Could you check a few things on this drawing? It's one solid part, dimensions in mm from its lowest x, y, z. A direction names the side the tool comes from. Round coordinates to 2 decimals unless told otherwise and drop trailing zeros. Write each loop counter-clockwise with the first axis right and the second up, starting at its lowest first coordinate (ties: lowest second). Pieces come first, ordered by that corner, then holes. Notation, with made-up numbers: (88.5, 70.25) -> (137.5, 70.25) arc R14 cw to (137.5, 75.25) -> close; hole circle Ø1 at (10.25, -27). An arc over 180 degrees is marked (long way). Answer in a Markdown table with one row per item. Add a question column.
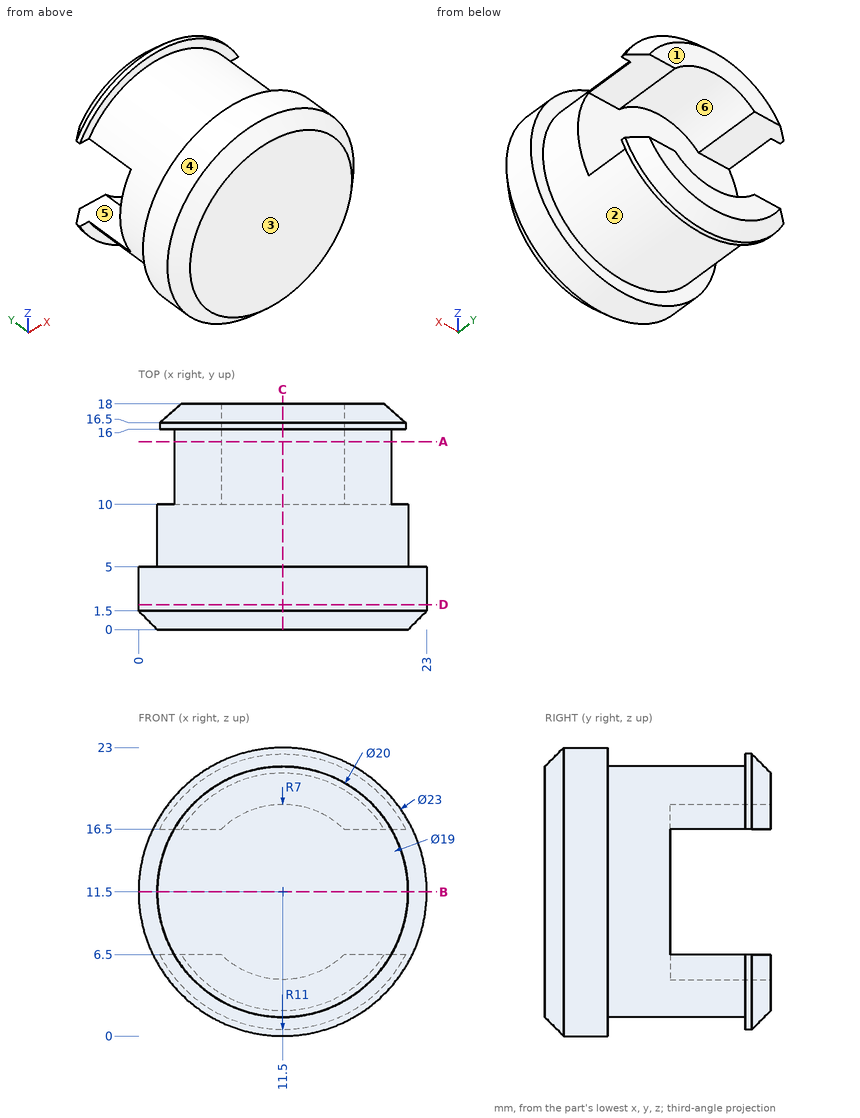
Item 1: If we section it at B-B on z = 11.5: Please give me the cut outline in (x, y), then the cut area to 3 significant figures.
Item 2: On a 3-axis mill with a long thin cutter (end or side, diameter ignored), from which of +Z, -Z, +X, -X, +Y, -Y can I reach the whole of each face in a straight line? I mean the marked faces 4, 5 and 6. Say none if no direction works.
Item 3: If we mould it in two halves opening along Y, with no side actions, what happens to the marked faces 1, 2 and 3? For each: pulls with the +Y half, pulls with the -Y half, needs draft (parallel to the pull), parting line crosses it, or undercut.
Item 4: For P1, Ø2, axis at x = 5, y = 13, coming from the -Z side; P2, Ø5.5, axis at x = 20, y = 13, coming from the -Z side; P3, Ø5.5, axis at x = 18.5, y = 14.5, coming from the +Z side; P4, Ø2, axis at y = 12, z = 10.5, coming from the +X side (3 decimals), each with a flat end and sliding along its axis, tell me the tip position at first contact or that it passes through.
Item 5: If we section it at D-D on y = 2: Please give me the cut outline in (x, z).
Item 6: If we section it at C-C on x = 11.5: Please give me the cut outline in (y, z).
Item 7: I need wall thicknesses on line 1 along X through (y, z) = (8.25, 9.5); line 2 along Y through (x, z) = (3, 18.25); line 3 along Y through (x, z) = (10.25, 12). Which ranges of each line are inside material? Lowest first, please. Write a range as from..to.
Item 8: If we section it at A-A on y = 15: Please give me the cut outline in (x, z).
Results list:
| question | item | result |
|---|---|---|
| 1 | outline | (0, 1.5) -> (1.5, 0) -> (21.5, 0) -> (23, 1.5) -> (23, 5) -> (21.5, 5) -> (21.5, 10) -> (1.5, 10) -> (1.5, 5) -> (0, 5) -> close |
| 1 | area | 213 mm² |
| 2 | face 4 | +Y, -Y |
| 2 | face 5 | +X, -X, +Y |
| 2 | face 6 | +Y |
| 3 | face 1 | pulls with the +Y half |
| 3 | face 2 | undercut |
| 3 | face 3 | pulls with the -Y half |
| 4 | P1 | z = 3.15 |
| 4 | P2 | z = 3.32 |
| 4 | P3 | z = 21.45 |
| 4 | P4 | through |
| 5 | outline | circle Ø23 at (11.5, 11.5) |
| 6 | outline | (0, 1.5) -> (1.5, 0) -> (5, 0) -> (5, 1.5) -> (16, 1.5) -> (16, 0.5) -> (16.5, 0.5) -> (18, 2) -> (18, 4.5) -> (10, 4.5) -> (10, 18.5) -> (18, 18.5) -> (18, 21) -> (16.5, 22.5) -> (16, 22.5) -> (16, 21.5) -> (5, 21.5) -> (5, 23) -> (1.5, 23) -> (0, 21.5) -> close |
| 7 | line 1 | 1.7..21.3 |
| 7 | line 2 | 0.85..5, 16..16.65 |
| 7 | line 3 | 0..10 |
| 8 | outline | (2.84, 6.5) arc R10 ccw to (20.16, 6.5) -> (16.4, 6.5) arc R7 cw to (6.6, 6.5) -> close; (2.84, 16.5) -> (6.6, 16.5) arc R7 cw to (16.4, 16.5) -> (20.16, 16.5) arc R10 ccw to start |
